Part print with two shaded views. Sizes in mm from the minimum x, y, z corner. A direction names the side the tool comes from. Give positions to 0.01 mm unless a question says otherwise; leave off trailing zeros. Write each loop counter-clockwise with the first axis right and the second up, starting at its lowest first coordinate (ties: lowest second). Pieces come first, ordered by that corner, then holes. Notation, with made-up numbers: (34, 82.5) - (52, 82.5) arc R22 ccw to (52, 102.5) - close; hole circle Ø2 at (89.5, 70). An arc over 180 degrees is marked (long way). One line per item, written item: value. Start each with the question number.
(1) 3-axis set-ups, long thin cutter, end or side, ignore diameter. For the marked faces 1, 2 and 3: which of +Z, -Z, +X, -X, +Y, -Y reach the whole face in a straight line?
(2) Cut at B-B, the plane x = 54.5. List the corners of the cut face in (y, z), and give its area (3 significant figures).
(3) Probe L1, parallel to Z at x = 30.5, y = 18; L2, parallel to X at y = 13, z = 11.75. List the from-to ranges inside material, lowest first.
(4) Cut at C-C, the plane y = 8. List the corners of the cut face in (x, z).
(5) Cut at D-D, the plane y = 26. List the corners of the cut face in (x, z).
(6) Cut at A-A, the plane z = 26.75. List the corners of the cut face in (x, y), and give its area (3 significant figures).
(7) Drop flat-ended pins along their axis: P1, Ø12, axis at x = 41, z = 6.5, coming from the +Y side; P2, Ø7.5, axis at y = 35, z = 14, coming from the +X side; P3, Ø1.1, axis at x = 8, y = 26, coming from the +Z side. Give the stop position or say it passes through.
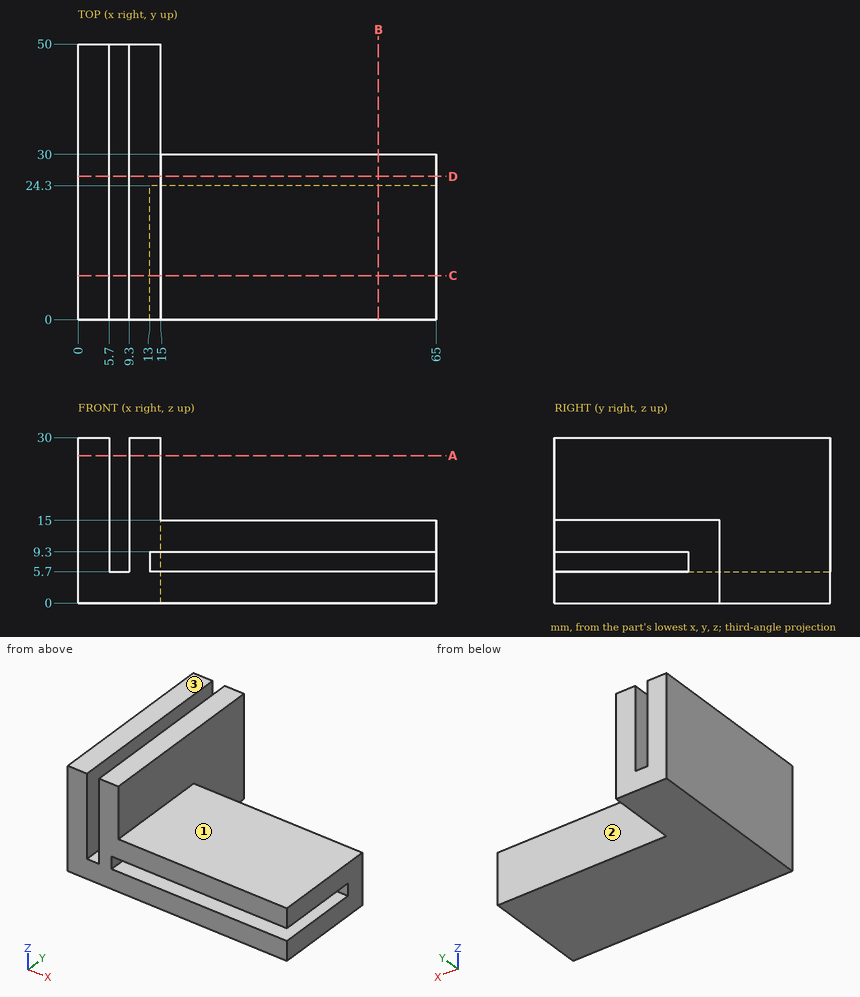
Answers follow:
1. face 1: +Z, +X, +Y, -Y
1. face 2: +Z, -Z, +X, +Y
1. face 3: +Z, +X, -X, +Y, -Y
2. outline: (0, 0) - (30, 0) - (30, 15) - (0, 15) - (0, 9.3) - (24.3, 9.3) - (24.3, 5.7) - (0, 5.7) - close
2. area: 363 mm²
3. L1: z = 0 to 5.7, 9.3 to 15
3. L2: x = 0 to 5.7, 9.3 to 65
4. outline: (0, 0) - (65, 0) - (65, 5.7) - (13, 5.7) - (13, 9.3) - (65, 9.3) - (65, 15) - (15, 15) - (15, 30) - (9.3, 30) - (9.3, 5.7) - (5.7, 5.7) - (5.7, 30) - (0, 30) - close
5. outline: (0, 0) - (65, 0) - (65, 15) - (15, 15) - (15, 30) - (9.3, 30) - (9.3, 5.7) - (5.7, 5.7) - (5.7, 30) - (0, 30) - close
6. outline: (0, 0) - (5.7, 0) - (5.7, 50) - (0, 50) - close; (9.3, 0) - (15, 0) - (15, 50) - (9.3, 50) - close
6. area: 570 mm²
7. P1: stops at y = 30
7. P2: stops at x = 15
7. P3: stops at z = 5.7
